Design review of the part shown in the three views and the two pictorial views. Dimensions are in mm from the part's minimum x, y and z. A direction names the side the tool comes from. Round coordinates to 2 decimals unless told otherwise and drop trailing zeros. Loops run counter-clockwise (first coordinate to the right, second up) from the corner with the lowest first, then second, coordinate; pieces in that order, holes last. Notation, with made-up numbers: (-19, 11) -> (-15, 11) arc R17 cw to (-15, 22) -> close; hole circle Ø2 at (5.5, -10.75). An arc over 180 degrees is marked (long way). Return JSON: item names as keys, results as strings. Group by question number.
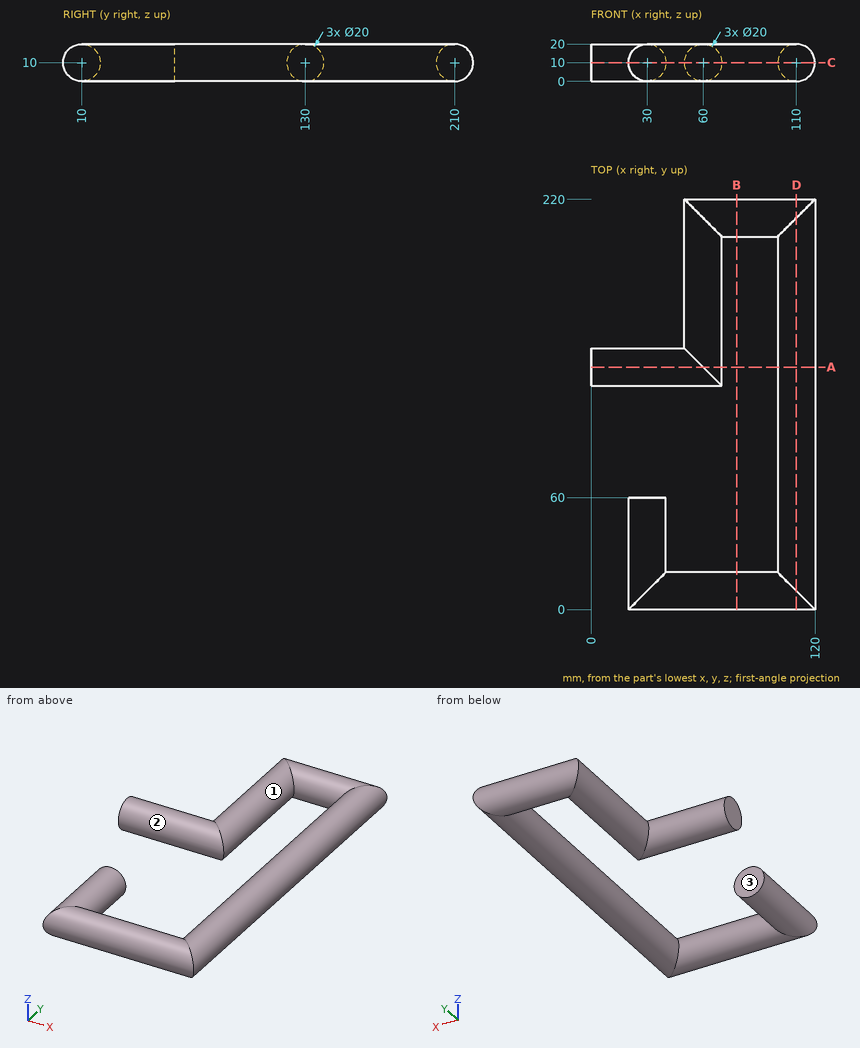
1. For P1, Ø1, axis at x = 58, z = 2.5, coming from the -Y side; P2, Ø8, axis at x = 23, z = 17, coming from the +Y side; P3, Ø6, axis at y = 60, z = 3.5, coming from the +X side, all flat-tipped, find the tip position at first contact; note any pin that passes through.
2. We need section B-B, the plane x = 78. Write out the cut boundary in (y, z), then the cut area to 3 significant figures.
3. Tool access review of the marked faces 1, 2 and 3: name each direction out of +Z, -Z, +X, -X, +Y, -Y from which nothing blocks a thin tool from reaching the whole face with its end or side.
4. We need section A-A, the plane y = 130. Write out the cut boundary in (x, z).
5. We need section D-D, the plane x = 110. Write out the cut boundary in (y, z), then the cut area to 3 significant figures.
6. Wall thickness on line 1 (Y direction, x = 45, z = 9.75); line 2 (X direction, y = 132, z = 9.75); line 3 (Y direction, x = 21, z = 13.5): over which ranges is each line inside the solid? List them lowest first.
7. We need section C-C, the plane z = 10. Write out the cut boundary in (x, y).
Check sheet entries:
{
 "1": {"P1": "stops at y = 2.86", "P2": "stops at y = 139.54", "P3": "stops at x = 119.37"},
 "2": {"outline": "circle Ø20 at (10, 10); circle Ø20 at (210, 10)", "area": "628 mm²"},
 "3": {"face 1": "none", "face 2": "-X", "face 3": "+Z, -Z, -X"},
 "4": {"outline": "(0, 0) -> (60, 0) arc R10 ccw to (60, 20) -> (0, 20) -> close; circle Ø20 at (110, 10)"},
 "5": {"outline": "(10, 0) -> (210, 0) arc R10 ccw to (210, 20) -> (10, 20) arc R10 ccw to start", "area": "4,310 mm²"},
 "6": {"line 1": "y = 0 to 20, 120 to 140", "line 2": "x = 0 to 70, 100 to 120", "line 3": "y = 0.63 to 60, 120.63 to 139.37"},
 "7": {"outline": "(0, 120) -> (70, 120) -> (70, 200) -> (100, 200) -> (100, 20) -> (40, 20) -> (40, 60) -> (20, 60) -> (20, 0) -> (120, 0) -> (120, 220) -> (50, 220) -> (50, 140) -> (0, 140) -> close"}
}
